```python
from build123d import *

# Parameters (mm, degrees)
CROQUIS1_R              = 8.9
CROQUIS1_R_2            = 2.5
SALIENTE_EXTRUIR1_DEPTH = 8.6
CROQUIS2_R              = 7
CROQUIS2_R_2            = 2.5
SALIENTE_EXTRUIR2_DEPTH = 1
CROQUIS3_R              = 6
CROQUIS3_R_2            = 2.5
SALIENTE_EXTRUIR3_DEPTH = 7
CROQUIS4_R              = 7
CROQUIS4_R_2            = 2.5
SALIENTE_EXTRUIR4_DEPTH = 1
CORTAR_EXTRUIR1_DEPTH   = 9.6


with BuildPart() as part:
    # Croquis1 → Saliente-Extruir1 (new body)
    with BuildSketch(Plane(origin=(0, 0, 0), x_dir=(1, 0, 0), z_dir=(0, 1, 0))):
        Circle(CROQUIS1_R)
        Circle(CROQUIS1_R_2, mode=Mode.SUBTRACT)
    extrude(amount=SALIENTE_EXTRUIR1_DEPTH)

    # Croquis2 → Saliente-Extruir2 (add)
    with BuildSketch(Plane(origin=(0, 8.6, 0), x_dir=(1, 0, 0), z_dir=(0, 1, 0))):
        Circle(CROQUIS2_R)
        Circle(CROQUIS2_R_2, mode=Mode.SUBTRACT)
    extrude(amount=SALIENTE_EXTRUIR2_DEPTH)

    # Croquis3 → Saliente-Extruir3 (add)
    with BuildSketch(Plane(origin=(0, 9.6, 0), x_dir=(1, 0, 0), z_dir=(0, 1, 0))):
        Circle(CROQUIS3_R)
        Circle(CROQUIS3_R_2, mode=Mode.SUBTRACT)
    extrude(amount=SALIENTE_EXTRUIR3_DEPTH)

    # Croquis4 → Saliente-Extruir4 (add)
    with BuildSketch(Plane(origin=(0, 16.6, 0), x_dir=(1, 0, 0), z_dir=(0, 1, 0))):
        Circle(CROQUIS4_R)
        Circle(CROQUIS4_R_2, mode=Mode.SUBTRACT)
    extrude(amount=SALIENTE_EXTRUIR4_DEPTH)

    # Croquis7 → Cortar-Extruir1 (cut, through all)
    with BuildSketch(Plane(origin=(0, 8.6, 0), x_dir=(1, 0, 0), z_dir=(0, 1, 0))):
        with BuildLine():
            Line((3.299612335, -8.265746091), (3.585413018, -6.433391848))
            Line((3.585413018, -6.433391848), (4.715491895, -7.548121368))
            ThreePointArc((4.715491895, -7.548121368), (4.023583013, -7.938562826), (3.299612335, -8.265746091))
        make_face()
    extrude(amount=-CORTAR_EXTRUIR1_DEPTH, mode=Mode.SUBTRACT)


solid = part.part
```
The model under review builds one solid part; all positions refer to its coordinate system, in mm. A direction names the side the tool comes from. Round coordinates to 2 decimals unless told otherwise and drop trailing zeros. Order: outer loops, then holes, each group sorted by start corner. A loop starts at its lowest first (then second) coordinate and runs counter-clockwise, first axis right, second up. Notation, with made-up numbers: (12.25, 0.5) - (21.25, 0.5) arc R9 cw to (21.25, 11.5) - close; hole circle Ø8 at (68, -19). An arc over 180 degrees is marked (long way). Answer in a Markdown table with one row per item.
(1) Clearance check with flat-ended pins moving along their axes: P1, Ø1.5, axis at x = -2.5, y = 2.5, coming from the -Z side; P2, Ø1, axis at y = 12, z = 2.5, coming from the +X side; P3, Ø6, axis at x = 5.5, y = 5, coming from the -Z side. State where each tip first meets the part, or that it passes through.
Result set:
| item | result |
|---|---|
| P1 | stops at z = -8.73 |
| P2 | stops at x = 5.66 |
| P3 | stops at z = -8.54 |
(2) Machinability: for faces 1 (the face through (3.44, 4.36, 7.36)), 2 (the face through (2, 0, 2)), 3 (the face through (6, 9.6, -2)), 4 (the face through (6.466, 9.093, 2.681)), 5 (the face through (0, 17.6, 3)), which of the approach directions +Z, -Z, +X, -X, +Y, -Y give a long, thin tool a straight path to every point of the face, cutting with its end or side? Answer none if there is none.
Result set:
| item | result |
|---|---|
| face 1 | +Z, +Y, -Y |
| face 2 | +Z, -Z, +X, -X, -Y |
| face 3 | none |
| face 4 | +Y |
| face 5 | +Z, -Z, +X, -X, +Y |
(3) Mouldability with a two-part tool opening along Z and no side actions: class faces 6 (the face through (-0.54, 8.68, 2.44)), 7 (the face through (-3, 8.6, -7)), 8 (the face through (-3.681, 4.24, -8.103)), 9 (the face through (4.14, 4.36, 6.98)) as released by +Z, released by -Z, zero draft, split by the parting line, or undercut.
Result set:
| item | result |
|---|---|
| face 6 | undercut |
| face 7 | zero draft |
| face 8 | split by the parting line |
| face 9 | released by +Z |
(4) For line 1 (Y direction, x = -5.25, z = 4.25); line 2 (X direction, y = 6.75, z = 0); line 3 (X direction, y = 11.25, z = 0), list the stretches that pass through material, from the lowest coordinate up. Write a range as from..to.
Result set:
| item | result |
|---|---|
| line 1 | y = 0..9.6, 16.6..17.6 |
| line 2 | x = -8.9..-2.5, 2.5..8.9 |
| line 3 | x = -6..-2.5, 2.5..6 |
(5) Take a section at D-D on z = -4.5. Write out the cut boundary in (x, y).
Result set:
| item | result |
|---|---|
| outline | (-7.68, 0) - (7.68, 0) - (7.68, 8.6) - (5.36, 8.6) - (5.36, 9.6) - (3.97, 9.6) - (3.97, 16.6) - (5.36, 16.6) - (5.36, 17.6) - (-5.36, 17.6) - (-5.36, 16.6) - (-3.97, 16.6) - (-3.97, 9.6) - (-5.36, 9.6) - (-5.36, 8.6) - (-7.68, 8.6) - close |
(6) Take a section at B-B on z = 0. Write out the cut boundary in (x, y).
Result set:
| item | result |
|---|---|
| outline | (-8.9, 0) - (-2.5, 0) - (-2.5, 17.6) - (-7, 17.6) - (-7, 16.6) - (-6, 16.6) - (-6, 9.6) - (-7, 9.6) - (-7, 8.6) - (-8.9, 8.6) - close; (2.5, 0) - (8.9, 0) - (8.9, 8.6) - (7, 8.6) - (7, 9.6) - (6, 9.6) - (6, 16.6) - (7, 16.6) - (7, 17.6) - (2.5, 17.6) - close |
(7) Take a section at C-C on y = 5.75. Write out the cut boundary in (x, z), plus the area to 3 significant figures.
Result set:
| item | result |
|---|---|
| outline | (3.3, 8.27) arc R8.9 ccw (long way) to (4.72, 7.55) - (3.59, 6.43) - close; hole circle Ø5 at (0, 0) |
| area | 228 mm2 |
(8) Take a section at A-A on x = 0. Write out the cut boundary in (y, z), plus the area to 3 significant figures.
Result set:
| item | result |
|---|---|
| outline | (0, -8.9) - (8.6, -8.9) - (8.6, -7) - (9.6, -7) - (9.6, -6) - (16.6, -6) - (16.6, -7) - (17.6, -7) - (17.6, -2.5) - (0, -2.5) - close; (0, 2.5) - (17.6, 2.5) - (17.6, 7) - (16.6, 7) - (16.6, 6) - (9.6, 6) - (9.6, 7) - (8.6, 7) - (8.6, 8.9) - (0, 8.9) - close |
| area | 177 mm2 |
